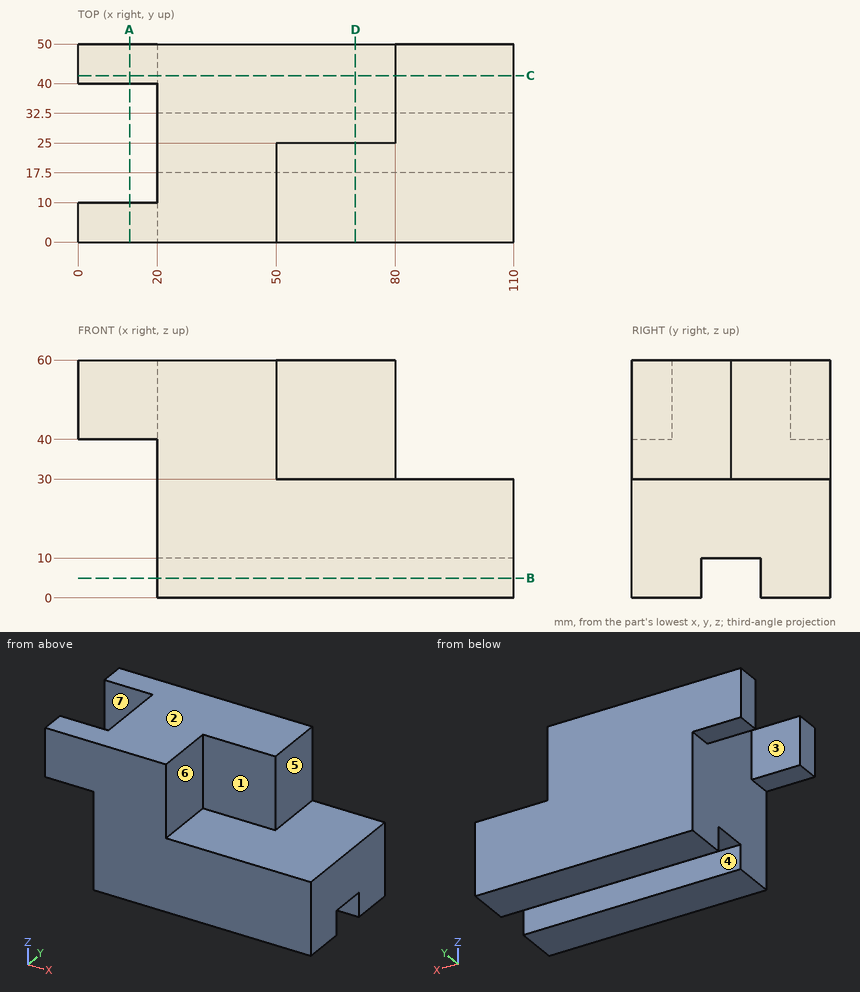
Geometry check sheet. Reference: drawing and pictorial views, mm from the part's lowest x, y, z. A direction names the side the tool comes from. Give positions to 0.01 mm unless a question says otherwise; leave off trailing zeros. Order: outer loops, then holes, each group sorted by start corner. A loop starts at its lowest first (then second) coordinate and runs counter-clockwise, first axis right, second up. Notation, with made-up numbers: M 85.5,68.5 L 104.5,68.5 A34 cw 104.5,98.5 Z; hole C 76,17 d5. An arc over 180 degrees is marked long. Answer in a Markdown table with one row per item.
1) Gauge pin test, flat ends, axial feed: P1, Ø8, axis at x = 10.5, y = 5.5, coming from the -Z side; P2, Ø20, axis at y = 10.5, z = 42, coming from the +X side; P3, Ø20, axis at y = 36.5, z = 43.5, coming from the +X side. Record the tip position at first contact, or that the pin passes through.
Filled sheet:
| item | result |
|---|---|
| P1 | stops at z = 40 |
| P2 | stops at x = 50 |
| P3 | stops at x = 80 |
2) Cross-section at B-B, the plane z = 5. Enter the section's corners in (x, y).
Filled sheet:
| item | result |
|---|---|
| outline | M 20,0 L 110,0 L 110,17.5 L 20,17.5 Z; M 20,32.5 L 110,32.5 L 110,50 L 20,50 Z |
3) Cross-section at A-A, the plane x = 13. Enter the section's corners in (y, z), plus the area to 3 significant figures.
Filled sheet:
| item | result |
|---|---|
| outline | M 0,40 L 10,40 L 10,60 L 0,60 Z; M 40,40 L 50,40 L 50,60 L 40,60 Z |
| area | 400 mm2 |
4) Release check for a two-part mould opening along Y. For the marked faces 1, 2 and 3 record: +Y half, -Y half, draft (parallel to the pull), parting line (faces both ways), or undercut.
Filled sheet:
| item | result |
|---|---|
| face 1 | -Y half |
| face 2 | draft |
| face 3 | undercut |
5) Thickness scan on L1, parallel to Y at x = 94.5, z = 9.5; L2, parallel to X at y = 13.5, z = 52.5; L3, parallel to X at y = 37, z = 17.5. Record the ranges inside material, lowest first. Write a range as [from, to].
Filled sheet:
| item | result |
|---|---|
| L1 | y = [0, 17.5], [32.5, 50] |
| L2 | x = [20, 50] |
| L3 | x = [20, 110] |
6) Access from +Z, -Z, +X, -X, +Y, -Y to the whole of each face (thin tool, end or side, straight path). Record for the marked faces 4, 5, 6 and 7.
Filled sheet:
| item | result |
|---|---|
| face 4 | -Z, +X, -X |
| face 5 | +Z, +X, +Y, -Y |
| face 6 | +Z, +X, -Y |
| face 7 | +Z, -Z, -X |
7) Cross-section at C-C, the plane y = 42. Enter the section's corners in (x, z).
Filled sheet:
| item | result |
|---|---|
| outline | M 0,40 L 20,40 L 20,0 L 110,0 L 110,30 L 80,30 L 80,60 L 0,60 Z |
8) Cross-section at D-D, the plane x = 70. Enter the section's corners in (y, z).
Filled sheet:
| item | result |
|---|---|
| outline | M 0,0 L 17.5,0 L 17.5,10 L 32.5,10 L 32.5,0 L 50,0 L 50,60 L 25,60 L 25,30 L 0,30 Z |
